Source: CAD feature listing. Evaluate the final solid. Frame: model axes, mm. A direction names the side the tool comes from. Round coordinates to 2 decimals unless told otherwise and drop trailing zeros. Order: outer loops, then holes, each group sorted by start corner. A loop starts at its lowest first (then second) coordinate and runs counter-clockwise, first axis right, second up. Notation, with made-up numbers: M 55,4 L 90,4 A34 ccw 90,41 Z; hole C -6,73 d9. An arc over 180 degrees is marked long. Answer as CSV lines item,"result". Start each with the question number.
Item 1: Pull-direction query (Z, two-part tool) for faces 5 (the face through (-10.117, 2, 8)), 6 (the face through (-48.705, -1.802, 5.723)), 7 (the face through (-8.603, -3.604, 11.446)); classes: +Z half, -Z half, draft (parallel to the pull), parting line (faces both ways), or undercut.
Item 2: Line query: line 1 (Y direction, x = -21, z = 0); line 2 (X direction, y = 8, z = 5.75); line 3 (Y direction, x = -30.5, z = -5) (3 decimals). Output: solid intervals per line, ascending. Write a range as [from, to].
Item 3: First-contact query: P1, Ø5, axis at x = -45.5, z = 0, coming from the +Y side; P2, Ø7, axis at y = 0, z = 0, coming from the -X side; P3, Ø10, axis at x = -15.5, z = 8.5, coming from the +Y side; P4, Ø3, axis at x = -49.5, y = -3.5, coming from the -Z side. Flat tips, straight axial feed; report the tip coordinate or a pass-through.
Item 4: Set-up query: faces 1 (the face through (-80.117, 8, 4)), 2 (the face through (-43.15, 7.81, -1.73)), 3 (the face through (-7.117, 8, -4)), 4 (the face through (-78.603, -3.604, 11.446)). Return all of +Z, -Z, +X, -X, +Y, -Y with unobstructed straight access to the full face (end or side cutting, diameter ignored); none if empty.
Item 5: Section query A-A on x = -63.5. Return the cut outline in (y, z).
from build123d import *

# Parameters (mm, degrees)
CHAMFER1_SIZE = 0.5


with BuildPart() as part:
    # Sketch1 → Revolve1 (revolve)
    with BuildSketch(Plane.XY, mode=Mode.PRIVATE) as revolve1_sk:
        Polygon((-90.116565428, 8), (-80.116565428, 8), (-80.116565428, 12), (-77.116565428, 12), (-77.116565428, 8), (-10.116565428, 8), (-10.116565428, 12), (-7.116565428, 12), (-7.116565428, 8), (-6.116565428, 8), (-6.116565428, 6), (-90.116565428, 6), align=None)
    revolve(revolve1_sk.sketch.rotate(Axis((-123.692772778, 0, 0), (1, 0, 0)), 90), axis=Axis((-123.692772778, 0, 0), (1, 0, 0)))

    # Chamfer1
    chamfer1_edges = [part.edges().sort_by_distance(p)[0] for p in [
        (-7.116565428, 0, -12),
        (-10.116565428, 0, -12),
        (-77.116565428, 0, -12),
        (-80.116565428, 0, -12),
        (-80.116565428, 0, -8),
        (-90.116565428, 0, -8),
        (-6.116565428, 0, -8),
        (-7.116565428, 0, -8),
    ]]
    chamfer(chamfer1_edges, length=CHAMFER1_SIZE - 0.0001)  # a hair under: the kernel refuses the full size


solid = part.part
Results:
1,face 5,"draft"
1,face 6,"undercut"
1,face 7,"parting line"
2,line 1,"[-8, -6], [6, 8]"
2,line 2,"[-80.12, -77.12], [-10.12, -7.12]"
2,line 3,"[-6.245, -3.317], [3.317, 6.245]"
3,P1,"y = 8"
3,P2,"through"
3,P3,"y = 7.19"
3,P4,"z = -7.75"
4,face 1,"-X"
4,face 2,"none"
4,face 3,"+X"
4,face 4,"+X, -X"
5,outline,"C 0,0 d16; hole C 0,0 d12"
